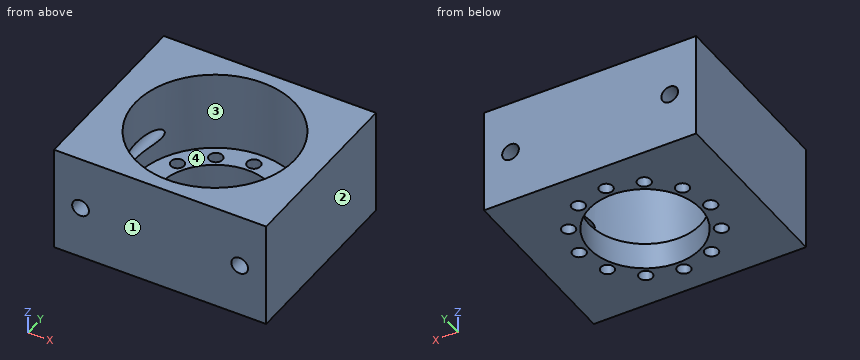
```python
from build123d import *

# Parameters (mm, degrees)
SKETCH1_W           = 50.8
SKETCH1_H           = 44.45
BOSS_EXTRUDE1_DEPTH = 25.4
SKETCH2_R           = 19.05
CUT_EXTRUDE1_DEPTH  = 19.05
SKETCH3_R           = 13.335
SKETCH3_R_2         = 1.5875
CUT_EXTRUDE2_DEPTH  = 71.138042459
SKETCH4_R           = 2
CUT_EXTRUDE3_DEPTH  = 73.122135992


with BuildPart() as part:
    # Sketch1 → Boss-Extrude1 (new body)
    with BuildSketch(Plane.XY):
        with Locations((25.4, 22.225)):
            Rectangle(SKETCH1_W, SKETCH1_H)
    extrude(amount=BOSS_EXTRUDE1_DEPTH)

    # Sketch2 → Cut-Extrude1 (cut)
    with BuildSketch(Plane.XY.offset(25.4)):
        with Locations((25.4, 22.225)):
            Circle(SKETCH2_R)
    extrude(amount=-CUT_EXTRUDE1_DEPTH, mode=Mode.SUBTRACT)

    # Sketch3 → Cut-Extrude2 (cut, through all)
    with BuildSketch(Plane.XY.offset(6.35)):
        with Locations((25.4, 22.225)):
            Circle(SKETCH3_R)
        with Locations((9.652, 22.225)):
            Circle(SKETCH3_R_2)
        with Locations((11.761831941, 30.099)):
            Circle(SKETCH3_R_2)
        with Locations((17.526, 35.863168059)):
            Circle(SKETCH3_R_2)
        with Locations((25.4, 37.973)):
            Circle(SKETCH3_R_2)
        with Locations((33.274, 35.863168059)):
            Circle(SKETCH3_R_2)
        with Locations((39.038168059, 30.099)):
            Circle(SKETCH3_R_2)
        with Locations((41.148, 22.225)):
            Circle(SKETCH3_R_2)
        with Locations((39.038168059, 14.351)):
            Circle(SKETCH3_R_2)
        with Locations((33.274, 8.586831941)):
            Circle(SKETCH3_R_2)
        with Locations((25.4, 6.477)):
            Circle(SKETCH3_R_2)
        with Locations((17.526, 8.586831941)):
            Circle(SKETCH3_R_2)
        with Locations((11.761831941, 14.351)):
            Circle(SKETCH3_R_2)
    extrude(amount=-CUT_EXTRUDE2_DEPTH, mode=Mode.SUBTRACT)

    # Sketch4 → Cut-Extrude3 (cut, through all)
    with BuildSketch(Plane(origin=(0, 44.45, 0), x_dir=(1, 0, 0), z_dir=(0, 1, 0))):
        with Locations(Location((6.35, -12.7, 0), (0, 0, 270))):
            Circle(SKETCH4_R)
        with Locations(Location((44.45, -12.7, 0), (0, 0, 270))):
            Circle(SKETCH4_R)
    extrude(amount=-CUT_EXTRUDE3_DEPTH, mode=Mode.SUBTRACT)


solid = part.part
```
The listing builds one solid part. Answer for the finished solid, in the listing's coordinates (mm). Face numbers are marked on the shaded views. Coordinates: 2 decimals unless noted, no trailing zeros. Loops run counter-clockwise (first coordinate to the right, second up) from the corner with the lowest first, then second, coordinate; pieces in that order, holes last. Notation, with made-up numbers: (-12, -36.75) -> (17, -36.75) arc R13 cw to (17, -25.75) -> close; hole circle Ø3 at (8, 84). An arc over 180 degrees is marked (long way). Use one line per item in the form item = value. Start each with the question number.
Item 1: The mould has two halves that part along X. Classify the marked faces 1, 2, 3 and 4: released by +X, released by -X, zero draft, split by the parting line, or undercut.
Item 2: The part is cut by section D-D on z = 8. Determine the outline of the cut face in (x, y) (3 decimals), then the cut area to 3 significant figures.
Item 3: The part is cut by section A-A on x = 25.4. Count the separate pieces of the cut face and the enclosed holes in it, then the cut area to 3 significant figures.
Item 4: Consider L1, parallel to Z at x = 6.35, y = 35; L2, parallel to Y at x = 24, z = 5.5; L3, parallel to X at y = 13, z = 12.5. Determine where each line is inside the solid, lowest interval first. Write a range as [from, to].
Item 5: The part is cut by section C-C on y = 26. Determine the outline of the cut face in (x, z).
Item 6: Flat-ended cylindrical pins translate along their axes: pin 1 Ø2.5 at (x, y) = (11.76, 30.1) entering from -Z; pin 2 Ø4 at (x, y) = (25.4, 37.973) entering from +Z. Find the tip coordinate at first contact, or state that the pin passes through.
Item 7: The part is cut by section B-B on z = 12.7. Determine the outline of the cut face in (x, y) (3 decimals), then the cut area to 3 significant figures.
Answer key:
q1.face_1 = zero draft
q1.face_2 = released by +X
q1.face_3 = undercut
q1.face_4 = undercut
q2.outline = (0, 0) -> (50.8, 0) -> (50.8, 44.45) -> (0, 44.45) -> close; hole circle Ø38.1 at (25.4, 22.225)
q2.area = 1,120 mm2
q3.separate_pieces = 4
q3.enclosed_holes = 0
q3.area = 194 mm2
q4.L1 = [0, 10.7], [14.7, 25.4]
q4.L2 = [0, 5.73], [7.23, 8.96], [35.49, 37.22], [38.72, 44.45]
q4.L3 = [0, 4.36], [8.34, 8.73], [42.07, 42.46], [46.44, 50.8]
q5.outline = (0, 0) -> (12.61, 0) -> (12.61, 6.35) -> (6.73, 6.35) -> (6.73, 10.74) arc R2 cw (long way) to (6.73, 14.66) -> (6.73, 25.4) -> (0, 25.4) -> close; (38.19, 0) -> (50.8, 0) -> (50.8, 25.4) -> (44.07, 25.4) -> (44.07, 14.66) arc R2 cw (long way) to (44.07, 10.74) -> (44.07, 6.35) -> (38.19, 6.35) -> close
q6.pin_1 = through
q6.pin_2 = 6.35
q7.outline = (0, 0) -> (4.35, 0) -> (4.35, 44.45) -> (0, 44.45) -> close; (8.35, 0) -> (42.45, 0) -> (42.45, 13.728) arc R19.05 cw to (8.35, 13.728) -> close; (8.35, 30.722) arc R19.05 cw to (42.45, 30.722) -> (42.45, 44.45) -> (8.35, 44.45) -> close; (46.45, 0) -> (50.8, 0) -> (50.8, 44.45) -> (46.45, 44.45) -> close
q7.area = 808 mm2
